Geometry: final body of the model. Coordinates: model frame, mm. Give positions to 0.01 mm unless a question says otherwise; leave off trailing zeros. Order: outer loops, then holes, each group sorted by start corner. A loop starts at its lowest first (then second) coordinate and runs counter-clockwise, first axis right, second up. Notation, with made-up numbers: (57.5, 57.25) - (114.5, 57.25) arc R23 cw to (114.5, 80.25) - close; hole circle Ø3 at (52, -36.75). An arc over 180 degrees is marked (long way). One line per item, written item: value.
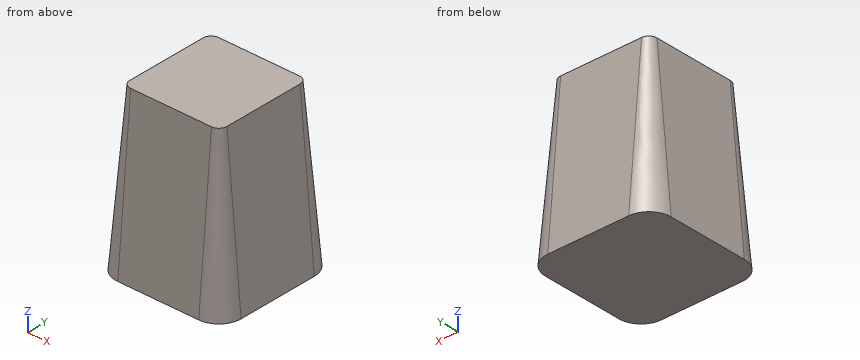
```python
from build123d import *

# Parameters (mm, degrees)
F1_DEPTH = 500
F1_TAPER = -5


with BuildPart() as f1:
    # F0 (on Top) → F1 (new body)
    with BuildSketch(Plane.XY):
        with BuildLine():
            ThreePointArc((-150, -125), (-142.6776695297, -142.6776695297), (-125, -150))
            Line((-125, -150), (125, -150))
            ThreePointArc((125, -150), (142.6776695297, -142.6776695297), (150, -125))
            Line((150, -125), (150, 125))
            ThreePointArc((150, 125), (142.6776695297, 142.6776695297), (125, 150))
            Line((125, 150), (-125, 150))
            ThreePointArc((-125, 150), (-142.6776695297, 142.6776695297), (-150, 125))
            Line((-150, 125), (-150, -125))
        make_face()
    extrude(amount=-F1_DEPTH, taper=F1_TAPER)


solid = f1.part
```
1) Material intervals for line 1 along Y through (x, z) = (-156.5, -212); line 2 along Y through (x, z) = (-125, -72); line 3 along X through (y, z) = (119.5, -150.5), sorted ascending.
Answers below:
line 1: -155.07 to 155.07
line 2: -156.3 to 156.3
line 3: -163.17 to 163.17
2) Section A-A, the plane z = -179. Return loops of the section in (x, y), then the cut area to 3 significant figures.
Answers below:
outline: (-165.66, -125) arc R40.66 ccw to (-125, -165.66) - (125, -165.66) arc R40.66 ccw to (165.66, -125) - (165.66, 125) arc R40.66 ccw to (125, 165.66) - (-125, 165.66) arc R40.66 ccw to (-165.66, 125) - close
area: 108,000 mm^2
3) First-contact query: pin 1 (10 mm diameter, centred on y = -108, z = -265.5, fed in from -X); pin 2 (10 mm diameter, centred on y = 115.5, z = -294, fed in from -X); pin 3 (8 mm diameter, centred on y = 52, z = -392, fed in from +X). Flat tips, straight axial feed; report the tip coordinate or a pass-through.
Answers below:
pin 1: x = -173.67
pin 2: x = -176.16
pin 3: x = 184.65
4) Section B-B, the plane y = 86.5. Return loops of the section in (x, z).
Answers below:
outline: (-193.74, -500) - (193.74, -500) - (150, 0) - (-150, 0) - close
5) Section D-D, the plane z = -424. Return loops of the section in (x, y), then the cut area to 3 significant figures.
Answers below:
outline: (-187.1, -125) arc R62.1 ccw to (-125, -187.1) - (125, -187.1) arc R62.1 ccw to (187.1, -125) - (187.1, 125) arc R62.1 ccw to (125, 187.1) - (-125, 187.1) arc R62.1 ccw to (-187.1, 125) - close
area: 137,000 mm^2
